The figure shows three views and two pictorial views of one solid part (mm, origin at its lowest corner). Answer the questions. A direction names the side the tool comes from. Coordinates: 2 decimals unless noted, no trailing zeros. Loops run counter-clockwise (first coordinate to the right, second up) from the corner with the lowest first, then second, coordinate; pieces in that order, holes last. Notation, with made-up numbers: M 66,63.25 L 94,63.25 A26 ccw 94,96.25 Z; hole C 78.5,36 d7. An arc over 180 degrees is marked long. Answer as a JSON object with one key per item and string values. Group by question number.
1. A cutting plane is placed at B-B on y = 3.75. Give the vertices of the cut face in (x, z).
2. Straight lines are drawn through the part: L1, parallel to Y at x = 0.25, z = 2; L2, parallel to Z at x = 0.5, y = 8.75. For each, find the intervals that lie inside material, in ascending order.
3. A cutting plane is placed at C-C on z = 2.75. Give the vertices of the cut face in (x, y), and give its area (3 significant figures).
4. A cutting plane is placed at A-A on x = 0.6. Give the vertices of the cut face in (y, z).
5. For the marked faces 1 and 2, determine the directions among +Z, -Z, +X, -X, +Y, -Y from which every point of the face is accessible in a straight line to the end or side of a thin tool.
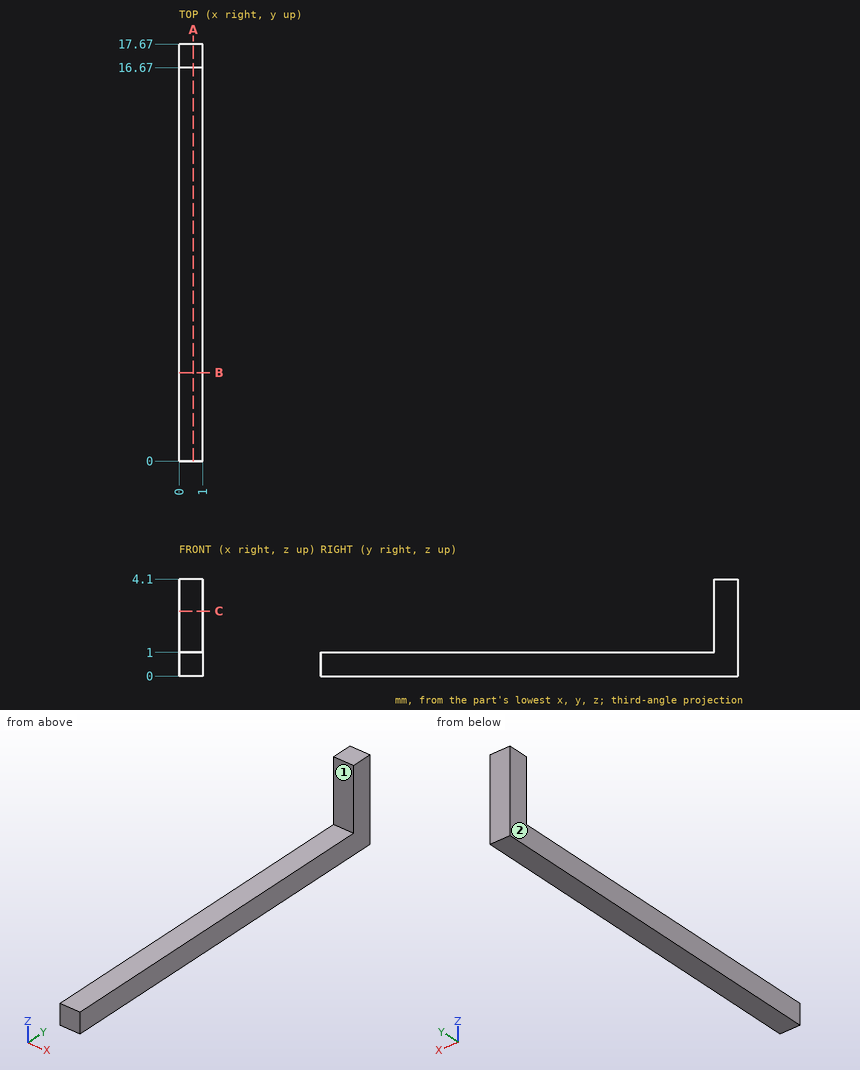
From the geometry:
{
 "1": {"outline": "M 0,0 L 1,0 L 1,1 L 0,1 Z"},
 "2": {"L1": "y = 16.67 to 17.67", "L2": "z = 0 to 1"},
 "3": {"outline": "M 0,16.67 L 1,16.67 L 1,17.67 L 0,17.67 Z", "area": "1.00 mm²"},
 "4": {"outline": "M 0,0 L 17.67,0 L 17.67,4.1 L 16.67,4.1 L 16.67,1 L 0,1 Z"},
 "5": {"face 1": "+Z, +X, -X, -Y", "face 2": "+Z, -Z, -X, +Y, -Y"}
}
